Input: part model. Units: mm. Frame: model coordinates. Coordinates: 2 decimals unless noted, no trailing zeros. Order: outer loops, then holes, each group sorted by start corner. A loop starts at its lowest first (then second) coordinate and runs counter-clockwise, first axis right, second up. Notation, with made-up numbers: (29, 70.5) -> (53, 70.5) arc R21 cw to (53, 76.5) -> close; hole circle Ø7 at (-11.5, 3.5). An arc over 180 degrees is marked (long way). Write each question's results on one line, items separated by ' | '.
```python
from build123d import *

# Parameters (mm, degrees)
F0_W     = 31.75
F0_H     = 82.55
F1_DEPTH = 31.75
F2_R     = 6.35
F4_DEPTH = 31.75


with BuildPart() as f1:
    # F0 (on Top) → F1 (new body)
    with BuildSketch(Plane.XY):
        with Locations((-15.875, 0)):
            Rectangle(F0_W, F0_H)
    extrude(amount=F1_DEPTH)

    # F2
    f2_edges = [f1.edges().sort_by_distance(p)[0] for p in [
        (0, 0, 0),
        (-31.75, 0, 0),
    ]]
    fillet(f2_edges, radius=F2_R)

    # F3 (on face) → F4 (cut)
    with BuildSketch(Plane.YZ):
        with BuildLine():
            ThreePointArc((-17.107905, -0.321605), (9.302694, -42.731185), (-0.278371, 6.302431))
            ThreePointArc((-0.278371, 6.302431), (-9.302694, 4.539097), (-17.107905, -0.321605))
        make_face()
    extrude(amount=-F4_DEPTH, mode=Mode.SUBTRACT)


solid = f1.part
```
(1) Cut plane B-B, the plane z = 4. Return loops of the section in (x, y) (3 decimals), plus the area to 3 significant figures.
Return value:
outline: (-31.299, -41.275) -> (-0.451, -41.275) -> (-0.451, -10.57) -> (-31.299, -10.57) -> close; (-31.299, 10.57) -> (-0.451, 10.57) -> (-0.451, 41.275) -> (-31.299, 41.275) -> close | area: 1,890 mm2
(2) Pin query (flat end, axial travel): P1, Ø1.5, axis at y = -22, z = 3.5, coming from the -X side. Return the tip coordinate at first contact, or that it passes through.
Return value:
P1: x = -31.39
(3) Cut plane D-D, the plane y = -8. Return loops of the section in (x, z).
Return value:
outline: (-31.75, 6.35) arc R6.35 ccw to (-31.61, 5.01) -> (-0.14, 5.01) arc R6.35 ccw to (0, 6.35) -> (0, 31.75) -> (-31.75, 31.75) -> close
(4) Line query: line 1 along Y through (x, z) = (-5, 3.5) (3 decimals); line 2 along Z through (x, y) = (-1, 1.5); line 3 along Z through (x, y) = (-6, -2.5). Output: solid intervals per line, ascending. Write a range as from..to.
Return value:
line 1: -41.275..-11.601, 11.601..41.275 | line 2: 6.26..31.75 | line 3: 6.18..31.75
(5) Cut plane C-C, the plane y = -28. Return loops of the section in (x, z).
Return value:
outline: (-31.75, 6.35) arc R6.35 ccw to (-25.4, 0) -> (-6.35, 0) arc R6.35 ccw to (0, 6.35) -> (0, 31.75) -> (-31.75, 31.75) -> close
(6) Cut plane A-A, the plane x = -15.5. Return loops of the section in (y, z) (3 decimals), plus the area to 3 significant figures.
Return value:
outline: (-41.275, 0) -> (-16.748, 0) arc R25.4 cw to (-0.278, 6.302) arc R25.4 cw to (16.748, 0) -> (41.275, 0) -> (41.275, 31.75) -> (-41.275, 31.75) -> close | area: 2,480 mm2
